Design review of the part shown in the three views and the two pictorial views. Dimensions are in mm from the part's minimum x, y and z. A direction names the side the tool comes from. Give positions to 0.01 mm unless a question says otherwise; leave off trailing zeros. Loops run counter-clockwise (first coordinate to the right, second up) from the corner with the lowest first, then second, coordinate; pieces in that order, holes last. Notation, with made-up numbers: (45.25, 66.25) - (87.25, 66.25) arc R9 ccw to (87.25, 82.25) - close; hole circle Ø5 at (84, -26.75). An arc over 180 degrees is marked (long way). Use CSV: the item, a comma, the result in double quotes. Start each with the question number.
1. Wall thickness on line 1 (X direction, y = 21, z = 2.5); line 2 (X direction, y = 45, z = 6.5); line 3 (Y direction, x = 12, z = 7.5): over which ranges is each line inside the solid? List them lowest first.
2. For the marked faces 1, 2 and 3, list the 3-axis set-ups (+Z, -Z, +X, -X, +Y, -Y) from which the entire face can be reached by the end or side of a thin tool; tool diameter is ignored.
3. For pin 1 (1 mm diameter, centred on y = 25.5, z = 8, fed in from +X); pin 2 (15 mm diameter, centred on x = 21.5, y = 25.5, fed in from +Z); pin 3 (0.8 mm diameter, centred on x = 29, z = 6.5, fed in from +Y), all flat-tipped, find the tip position at first contact; note any pin that passes through.
4. Take a section at B-B on x = 21. Give the boundary of the cut face in (y, z).
5. Take a section at A-A on y = 20. Give the boundary of the cut face in (x, z).
6. Take a section at D-D on z = 8.25. Give the boundary of the cut face in (x, y), plus the area to 3 significant figures.
7. Take a section at C-C on z = 1.25. Give the boundary of the cut face in (x, y).
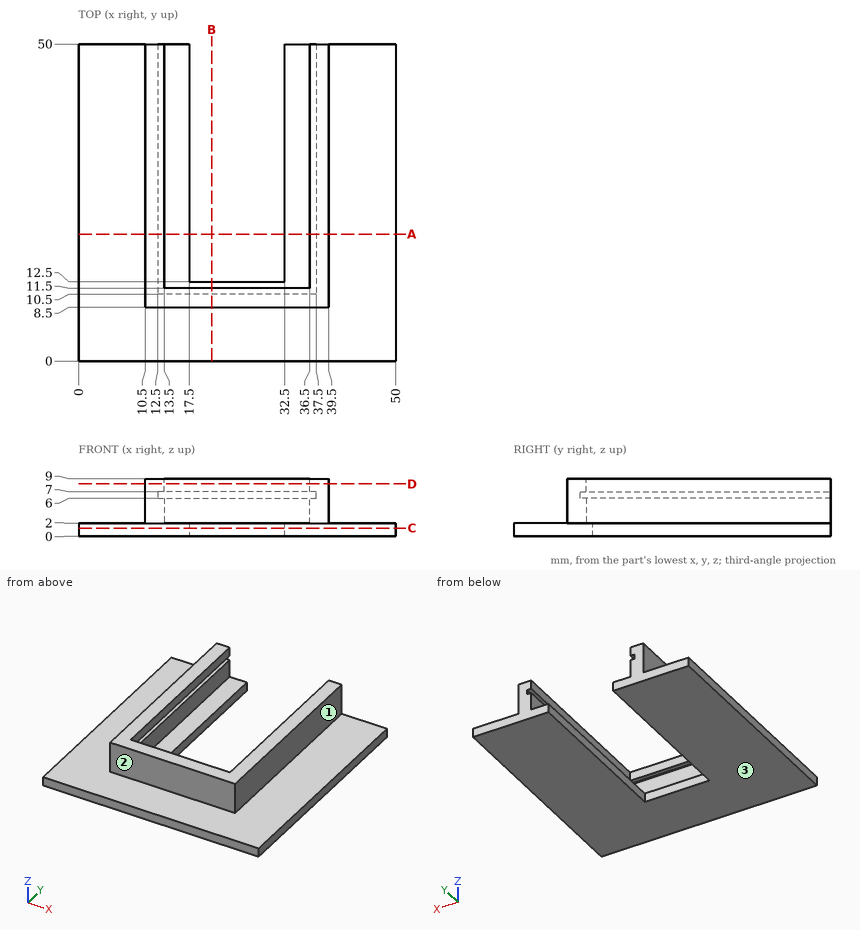
Check result:
1,line 1,"x = 10.5 to 13.5, 36.5 to 39.5"
1,line 2,"x = 10.5 to 12.5, 37.5 to 39.5"
1,line 3,"y = 8.5 to 50"
2,face 1,"+Z, +X, +Y, -Y"
2,face 2,"+Z, +X, -X, -Y"
2,face 3,"-Z, +X, -X, +Y, -Y"
3,pin 1,"stops at x = 39.5"
3,pin 2,"stops at z = 2"
3,pin 3,"stops at y = 10.5"
4,outline,"(0, 0) - (12.5, 0) - (12.5, 2) - (11.5, 2) - (11.5, 6) - (10.5, 6) - (10.5, 7) - (11.5, 7) - (11.5, 9) - (8.5, 9) - (8.5, 2) - (0, 2) - close"
5,outline,"(0, 0) - (17.5, 0) - (17.5, 2) - (13.5, 2) - (13.5, 6) - (12.5, 6) - (12.5, 7) - (13.5, 7) - (13.5, 9) - (10.5, 9) - (10.5, 2) - (0, 2) - close; (32.5, 0) - (50, 0) - (50, 2) - (39.5, 2) - (39.5, 9) - (36.5, 9) - (36.5, 7) - (37.5, 7) - (37.5, 6) - (36.5, 6) - (36.5, 2) - (32.5, 2) - close"
6,outline,"(10.5, 8.5) - (39.5, 8.5) - (39.5, 50) - (36.5, 50) - (36.5, 11.5) - (13.5, 11.5) - (13.5, 50) - (10.5, 50) - close"
6,area,"318 mm²"
7,outline,"(0, 0) - (50, 0) - (50, 50) - (32.5, 50) - (32.5, 12.5) - (17.5, 12.5) - (17.5, 50) - (0, 50) - close"
